Part print with two shaded views. Sizes in mm from the minimum x, y, z corner. Round coordinates to 2 decimals unless told otherwise and drop trailing zeros. Loops run counter-clockwise (first coordinate to the right, second up) from the corner with the lowest first, then second, coordinate; pieces in that order, holes last.
(1) Mould opens along Y. For the marked faces 1, 2 and 3 say: +Y half, -Y half, draft (parallel to the pull), parting line (faces both ways), or undercut.
(2) Cut at B-B on y = 6. List the corners of the cut face in (x, z).
(3) Flat gauge pins, fed straight in: pin 1 (12 mm diameter, centred on x = 6, z = 19, fed in from +Y); pin 2 (3.5 mm diameter, centred on x = 12, y = 14, fed in from +Z); pin 3 (4.5 mm diameter, centred on x = 20, z = 14, fed in from -Y); pin 4 (6.5 mm diameter, centred on x = 20, y = 14, fed in from +Z). Where does each tip first touch, or does it go through?
(4) Probe probe 1 along X at (y, z) = (1.5, 6); probe 2 along Y at (x, z) = (4, 0.55). List the from-to ranges inside material, lowest first.
(5) Cut at D-D on y = 17.25. List the corners of the cut face in (x, z).
(6) Cut at A-A on x = 20. Count the separate pieces of the cut face and the enclosed holes in it, then the cut area to 3 significant figures.
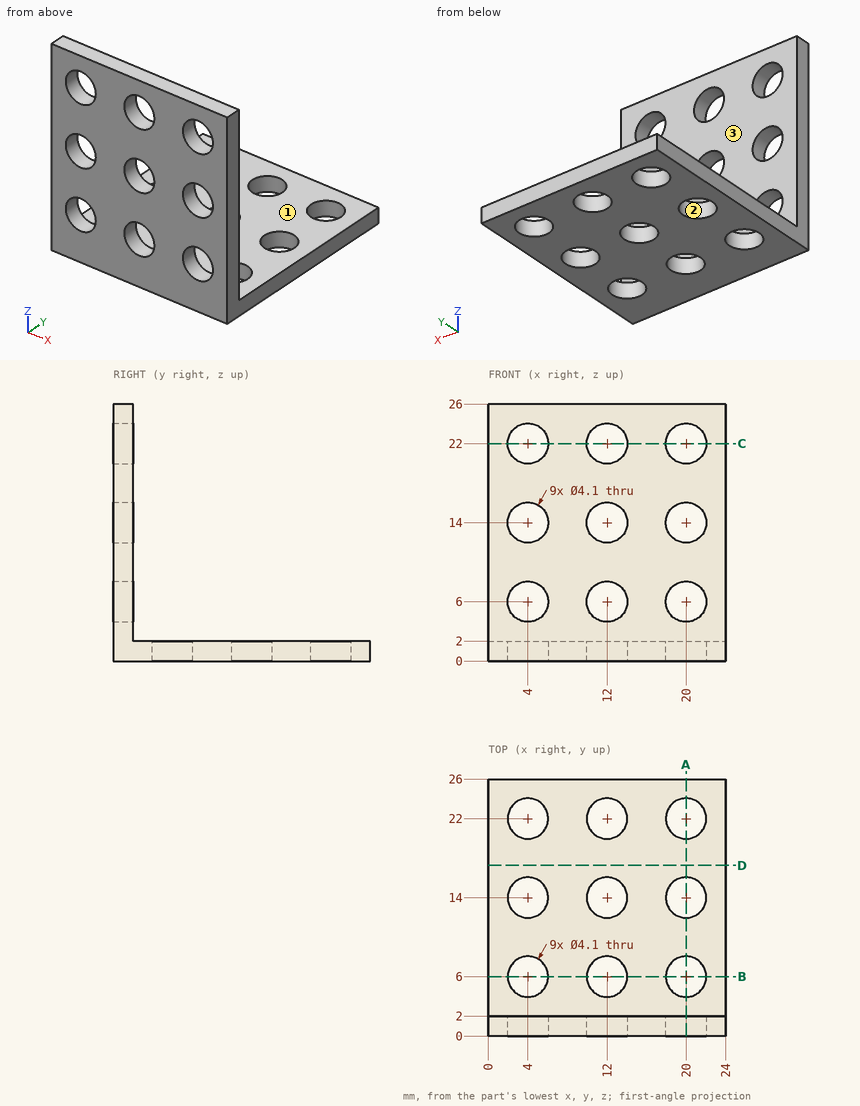
Final values:
1. face 1: draft
1. face 2: undercut
1. face 3: +Y half
2. outline: (0, 0) - (1.95, 0) - (1.95, 2) - (0, 2) - close; (6.05, 0) - (9.95, 0) - (9.95, 2) - (6.05, 2) - close; (14.05, 0) - (17.95, 0) - (17.95, 2) - (14.05, 2) - close; (22.05, 0) - (24, 0) - (24, 2) - (22.05, 2) - close
3. pin 1: stops at y = 2
3. pin 2: passes through
3. pin 3: stops at y = 0
3. pin 4: stops at z = 2
4. probe 1: x = 0 to 1.95, 6.05 to 9.95, 14.05 to 17.95, 22.05 to 24
4. probe 2: y = 0 to 3.95, 8.05 to 11.95, 16.05 to 19.95, 24.05 to 26
5. outline: (0, 0) - (24, 0) - (24, 2) - (0, 2) - close
6. separate pieces: 7
6. enclosed holes: 0
6. area: 50.8 mm2
